The listing builds one solid part. Answer for the finished solid, in the listing's coordinates (mm). Face numbers are marked on the shaded views. A direction names the side the tool comes from. Give positions to 0.01 mm unless a question says otherwise; leave off trailing zeros. Loops run counter-clockwise (first coordinate to the right, second up) from the corner with the lowest first, then second, coordinate; pieces in that order, holes last. Notation, with made-up numbers: (77.5, 79) - (119.5, 79) arc R19 ccw to (119.5, 91) - close; hole circle Ø4 at (49.5, 88). An arc over 180 degrees is marked (long way). One line per item, written item: value. Start each with the question number.
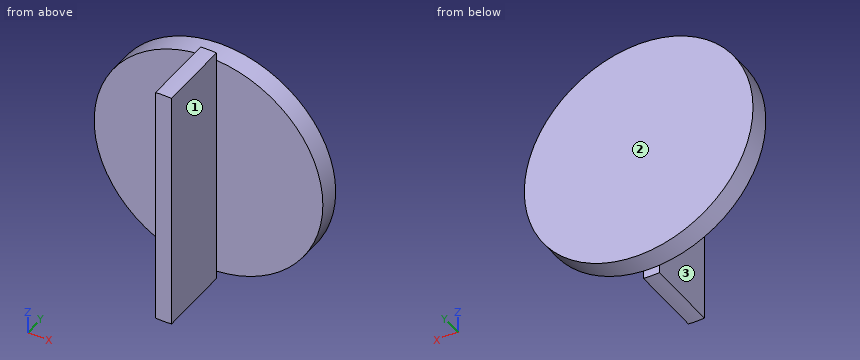
from build123d import *

# Parameters (mm, degrees)
F0_W     = 9.525
F0_H     = 145.739072
F2_DEPTH = 44.45
F1_R     = 68.2625
F3_DEPTH = 12.7


with BuildPart() as f2:
    # F0 (on Front) → F2 (new body)
    with BuildSketch(Plane.XZ):
        with BuildLine():
            Line((-4.7625, 72.869536), (4.7625, 72.869536))
            ThreePointArc((4.7625, 72.869536), (0, 73.025), (-4.7625, 72.869536))
        make_face()
        with BuildLine():
            ThreePointArc((-4.7625, -72.869536), (0, -73.025), (4.7625, -72.869536))
            Line((4.7625, -72.869536), (-4.7625, -72.869536))
        make_face()
        Rectangle(F0_W, F0_H)
    extrude(amount=F2_DEPTH)

    # F1 (on Front) → F3 (join)
    with BuildSketch(Plane.XZ):
        Circle(F1_R)
    extrude(amount=-F3_DEPTH)


solid = f2.part
1. Flat-ended cylindrical pins translate along their axes: pin 1 (3 mm diameter, centred on x = -6, y = -30.5, fed in from +Z); pin 2 (22 mm diameter, centred on y = -28, z = 31, fed in from +X); pin 3 (10 mm diameter, centred on x = -24.5, y = 6.5, fed in from -Z). Find the tip coordinate at first contact, or state that the pin passes through.
2. A cutting plane is placed at B-B (y = -22). Determine the outline of the cut face in (x, z).
3. Find the intervals of material crossed by L1, parallel to X at y = -18, z = 48.5; L2, parallel to Y at x = 26, z = -42; L3, parallel to Z at x = 46.5, y = 2, in increasing order. Write a range as [from, to].
4. A cutting plane is placed at A-A (z = 0). Determine the outline of the cut face in (x, y).
5. A cutting plane is placed at D-D (z = 29). Determine the outline of the cut face in (x, y).
6. For the marked faces 1, 2 and 3, determine the directions among +Z, -Z, +X, -X, +Y, -Y from which every point of the face is accessible in a straight line to the end or side of a thin tool.
7. A cutting plane is placed at C-C (x = -45). Determine the outline of the cut face in (y, z), plus the area to 3 significant figures.
Results below:
1. pin 1: stops at z = 72.89
1. pin 2: stops at x = 4.76
1. pin 3: stops at z = -65.42
2. outline: (-4.76, -72.87) arc R73.03 ccw to (4.76, -72.87) - (4.76, 72.87) arc R73.03 ccw to (-4.76, 72.87) - close
3. L1: x = [-4.76, 4.76]
3. L2: y = [0, 12.7]
3. L3: z = [-49.98, 49.98]
4. outline: (-68.26, 0) - (-4.76, 0) - (-4.76, -44.45) - (4.76, -44.45) - (4.76, 0) - (68.26, 0) - (68.26, 12.7) - (-68.26, 12.7) - close
5. outline: (-61.8, 0) - (-4.76, 0) - (-4.76, -44.45) - (4.76, -44.45) - (4.76, 0) - (61.8, 0) - (61.8, 12.7) - (-61.8, 12.7) - close
6. face 1: +Z, -Z, +X, -Y
6. face 2: +Z, -Z, +X, -X, +Y
6. face 3: +Z, -Z, -X, -Y
7. outline: (0, -51.33) - (12.7, -51.33) - (12.7, 51.33) - (0, 51.33) - close
7. area: 1,300 mm^2
